Autodesk Inventor part; units mm, degrees
ref_plane "YZ Plane" through (0, 0, 0) normal (1, 0, 0) x (0, 1, 0)
ref_plane "XZ Plane" through (0, 0, 0) normal (0, 1, 0) x (-1, 0, 0)
ref_plane "XY Plane" through (0, 0, 0) normal (0, 0, 1) x (1, 0, 0)
sketch "Sketch1" plane through (0, 0, 0) normal (0, 0, 1) x (1, 0, 0)
  line L0 (0, 0) -> (70, 0)
  line L1 (70, 0) -> (70, 22)
  line L2 (70, 22) -> (0, 22)
  line L3 (0, 22) -> (0, 0)
  dimension "d0" = 70
  dimension "d1" = 22
extrude "Extrusion1" add sketch "Sketch1" along normal blind 10
chamfer "Chamfer1" distance 4 angle 45 2 edges at (35, 22, 10) (35, 0, 10)
fillet "Fillet1" radius 0.5 12 edges at (35, 22, 6) (35, 18, 10) (70, 20, 8) (70, 22, 3) (70, 11, 10) (70, 2, 8) (70, 0, 3) (35, 4, 10) (0, 11, 10) (0, 2, 8) (0, 0, 3) (35, 0, 6)
properties part number "batt_cap" material "Glass"
Input: part model. Units: mm. Frame: model coordinates. Round coordinates to 2 decimals unless told otherwise and drop trailing zeros. Loops run counter-clockwise (first coordinate to the right, second up) from the corner with the lowest first, then second, coordinate; pieces in that order, holes last.
1) Pin query (flat end, axial travel): pin 1 (2 mm diameter, centred on x = 45.5, z = 4.5, fed in from -Y). Return the tip coordinate at first contact, or that it passes through.
Ans:
pin 1: stops at y = 0
2) Section query A-A on x = 6.5. Return the cut outline in (y, z).
Ans:
outline: (0, 0) - (22, 0) - (22, 5.79) arc R0.5 ccw to (21.85, 6.15) - (18.15, 9.85) arc R0.5 ccw to (17.79, 10) - (4.21, 10) arc R0.5 ccw to (3.85, 9.85) - (0.15, 6.15) arc R0.5 ccw to (0, 5.79) - close
3) Material intervals for line 1 (Z direction, x = 4.5, y = 20.5); line 2 (Z direction, x = 19, y = 20.25); line 3 (Y direction, x = 18, z = 8.75), sorted ascending.
Ans:
line 1: z = 0 to 7.5
line 2: z = 0 to 7.75
line 3: y = 2.75 to 19.25
